```python
from build123d import *

# Parameters (mm, degrees)
SKETCH2_R                 = 203
BOSS_EXTRUDE1_DEPTH       = 25
SKETCH3_R                 = 165
BOSS_EXTRUDE4_DEPTH       = 20
BOSS_EXTRUDE6_DEPTH       = 45
BOSS_EXTRUDE7_DEPTH       = 202.626802206
SKETCH12_W                = 400
SKETCH12_H                = 84
CUT_EXTRUDE2_DEPTH        = 195
SKETCH13_R                = 65
BOSS_EXTRUDE8_DEPTH       = 5
SKETCH14_R                = 59.5
BOSS_EXTRUDE9_DEPTH       = 14
SKETCH15_R                = 21.046280496
BOSS_EXTRUDE10_DEPTH      = 14
BOSS_EXTRUDE11_DEPTH      = 25
BOSS_EXTRUDE12_DEPTH      = 65
BOSS_EXTRUDE12_DEPTH_BACK = 25
BOSS_EXTRUDE13_DEPTH      = 25
BOSS_EXTRUDE13_DEPTH_BACK = 15
FILLET1_R                 = 10
SKETCH20_R                = 116.015
BOSS_EXTRUDE14_DEPTH      = 10


with BuildPart() as part:
    # Sketch2 → Boss-Extrude1 (new body)
    with BuildSketch(Plane(origin=(0, 0, 0), x_dir=(1, 0, 0), z_dir=(0, 1, 0))):
        with Locations(Location((0, 0, 0), (0, 0, 270))):
            Circle(SKETCH2_R)
    extrude(amount=BOSS_EXTRUDE1_DEPTH)

    # Sketch3 → Boss-Extrude4 (add)
    with BuildSketch(Plane(origin=(0, 25, 0), x_dir=(1, 0, 0), z_dir=(0, 1, 0))):
        with Locations(Location((0, 0, 0), (0, 0, 270))):
            Circle(SKETCH3_R)
    extrude(amount=BOSS_EXTRUDE4_DEPTH)

    # Sketch8 → Boss-Extrude6 (add)
    with BuildSketch(Plane(origin=(0, 45, 0), x_dir=(1, 0, 0), z_dir=(0, 1, 0))):
        Polygon((-36.218523686, 88.373197794), (-36.218523686, 142.845857418), (-66.931831772, 173.559165504), (-278.448010099, 88.373197794), (-278.448010099, -114.626802206), (-36.218523686, -114.626802206), align=None)
    extrude(amount=-BOSS_EXTRUDE6_DEPTH)

    # Sketch11 → Boss-Extrude7 (add)
    with BuildSketch(Plane.XY.offset(-88)):
        Polygon((-278.448010099, 0), (-364.82630567, -41.890214301), (-773.82630567, -41.890214301), (-773.82630567, 82.109785699), (-433.530139449, 82.109785699), (-278.448010099, 45), align=None)
    extrude(amount=BOSS_EXTRUDE7_DEPTH)

    # Sketch12 → Cut-Extrude2 (cut)
    with BuildSketch(Plane(origin=(0, 0, -88), x_dir=(-1, 0, 0), z_dir=(0, 0, -1))):
        with Locations((573.82630567, 20.109785699)):
            Rectangle(SKETCH12_W, SKETCH12_H)
    extrude(amount=-CUT_EXTRUDE2_DEPTH, mode=Mode.SUBTRACT)

    # Sketch13 → Boss-Extrude8 (add)
    with BuildSketch(Plane.XZ.offset(41.890214301)):
        with Locations((-572.873962689, 13.972710812)):
            Circle(SKETCH13_R)
    extrude(amount=BOSS_EXTRUDE8_DEPTH)

    # Sketch14 → Boss-Extrude9 (add)
    with BuildSketch(Plane.XZ.offset(46.890214301)):
        with Locations((-572.873962689, 13.972710812)):
            Circle(SKETCH14_R)
    extrude(amount=BOSS_EXTRUDE9_DEPTH)

    # Sketch15 → Boss-Extrude10 (add)
    with BuildSketch(Plane(origin=(0, 82.109785699, 0), x_dir=(1, 0, 0), z_dir=(0, 1, 0))):
        with Locations(Location((-702.441522293, -14.627430099, 0), (0, 0, 90))):
            Circle(SKETCH15_R)
        with Locations(Location((-628.892568706, -14.627430099, 0), (0, 0, 90))):
            Circle(SKETCH15_R)
        with Locations(Location((-572.1226233, -14.627430099, 0), (0, 0, 90))):
            Circle(SKETCH15_R)
    extrude(amount=BOSS_EXTRUDE10_DEPTH)

    # Sketch16 → Boss-Extrude11 (add)
    with BuildSketch(Plane(origin=(0, 96.109785699, 0), x_dir=(1, 0, 0), z_dir=(0, 1, 0))):
        with BuildLine():
            Line((-556.497428598, 64.069909455), (-974.176536307, 64.069909455))
            Line((-974.176536307, 64.069909455), (-1038.149417409, 0.097028353))
            ThreePointArc((-1038.149417409, 0.097028353), (-1064.162147568, -38.833773506), (-1073.296603667, -84.75578539))
            Line((-1073.296603667, -84.75578539), (-1073.296603667, -142.077234659))
            ThreePointArc((-1073.296603667, -142.077234659), (-1038.149417409, -226.930048402), (-953.296603667, -262.077234659))
            Line((-953.296603667, -262.077234659), (-636.497428598, -262.077234659))
            ThreePointArc((-636.497428598, -262.077234659), (-551.644614856, -226.930048402), (-516.497428598, -142.077234659))
            Line((-516.497428598, -142.077234659), (-516.497428598, 24.069909455))
            ThreePointArc((-516.497428598, 24.069909455), (-528.213157351, 52.354180702), (-556.497428598, 64.069909455))
        make_face()
    extrude(amount=BOSS_EXTRUDE11_DEPTH)

    # Sketch17 → Boss-Extrude12 (add, two sides: drawn at the far end of the back side and taken through both)
    with BuildSketch(Plane.ZY.offset(1073.296603667).offset(-BOSS_EXTRUDE12_DEPTH_BACK)):
        with BuildLine():
            Line((8.768612392, 544.923564191), (123.173449264, 544.923564191))
            ThreePointArc((123.173449264, 544.923564191), (222.16839863, 503.918513558), (263.173449264, 404.923564191))
            Line((263.173449264, 404.923564191), (263.173449264, -54.759891123))
            ThreePointArc((263.173449264, -54.759891123), (222.16839863, -153.754840489), (123.173449264, -194.759891123))
            Line((123.173449264, -194.759891123), (8.768612392, -194.759891123))
            ThreePointArc((8.768612392, -194.759891123), (-90.226336974, -153.754840489), (-131.231387608, -54.759891123))
            Line((-131.231387608, -54.759891123), (-131.231387608, 404.923564191))
            ThreePointArc((-131.231387608, 404.923564191), (-90.226336974, 503.918513558), (8.768612392, 544.923564191))
        make_face()
    extrude(amount=BOSS_EXTRUDE12_DEPTH + BOSS_EXTRUDE12_DEPTH_BACK)

    # Sketch19 → Boss-Extrude13 (add, two sides: drawn at the far end of the back side and taken through both)
    with BuildSketch(Plane(origin=(0, 0, -23.231387608), x_dir=(-1, 0, 0), z_dir=(0, 0, -1)).offset(-BOSS_EXTRUDE13_DEPTH_BACK)):
        Polygon((1052.931156926, -16.752524753), (985.063520649, 100.43883668), (1052.931156926, 100.43883668), align=None)
    extrude(amount=BOSS_EXTRUDE13_DEPTH + BOSS_EXTRUDE13_DEPTH_BACK)

    # Fillet1
    fillet1_edges = [part.edges().sort_by_distance(p)[0] for p in [
        (-1048.296603667, -8.749747053, -28.231387608),
        (-987.570552343, 96.109785699, -28.231387608),
    ]]
    fillet(fillet1_edges, radius=FILLET1_R)

    # Sketch20 → Boss-Extrude14 (add)
    with BuildSketch(Plane(origin=(-1048.296603667, 0, 0), x_dir=(0, 0, -1), z_dir=(1, 0, 0))):
        with Locations(Location((-39.49671875, 302.878292984, 0), (0, 0, 270))):
            Circle(SKETCH20_R)
    extrude(amount=BOSS_EXTRUDE14_DEPTH)


solid = part.part
```
The model under review builds one solid part; all positions refer to its coordinate system, in mm. A direction names the side the tool comes from. Round coordinates to 2 decimals unless told otherwise and drop trailing zeros. Loops run counter-clockwise (first coordinate to the right, second up) from the corner with the lowest first, then second, coordinate; pieces in that order, holes last. Notation, with made-up numbers: M 42.25,1 L 47.25,1 A24 cw 47.25,19 Z; hole C -1.5,64.5 d10. An arc over 180 degrees is marked long. Answer as a JSON object with one key per item and string values.
(1) Clearance check with flat-ended pins moving along their axes: P1, Ø20, axis at x = -806, y = 108, coming from the +Z side; P2, Ø8, axis at y = -91.5, z = 145, coming from the +X side; P3, Ø12.5, axis at y = 110, z = 59, coming from the +X side. State where each tip first meets the part, or that it passes through.
Resolved:
{"P1": "z = 262.08", "P2": "x = -1048.3", "P3": "x = -516.5"}
(2) Take a section at D-D on x = -815.5. Give the boundary of the cut face in (y, z).
Resolved:
{"outline": "M 96.11,-64.07 L 121.11,-64.07 L 121.11,262.08 L 96.11,262.08 Z"}
(3) Take a section at B-B on z = 233. Give the boundary of the cut face in (x, y), and give its area (3 significant figures).
Resolved:
{"outline": "M -1138.3,-141.58 L -1048.3,-141.58 L -1048.3,491.75 L -1138.3,491.75 Z; M -1031.61,96.11 L -558.18,96.11 L -558.18,121.11 L -1031.61,121.11 Z", "area": "68,800 mm²"}
(4) Take a section at A-A on x = 0. Give the boundary of the cut face in (y, z).
Resolved:
{"outline": "M 0,-203 L 25,-203 L 25,-165 L 45,-165 L 45,165 L 25,165 L 25,203 L 0,203 Z"}
(5) To check wall thickness, follow line 1 along Y through (x, z) = (-706.5, -62); line 2 along Y through (x, z) = (-713, 208); line 3 along X through (y, z) = (85, 219). State the ranges of each line that lie inside material, in increasing order.
Resolved:
{"line 1": "-41.89 to -21.89, 62.11 to 82.11, 96.11 to 121.11", "line 2": "96.11 to 121.11", "line 3": "-1138.3 to -1048.3"}
(6) Draft analysis for pull direction X (two halves, no side actions). For faces 6 (the flat face through (-516.497, 108, 60)), 7 (the flat face through (-467.6, 62.3, -88)), 8 (the flat face through (-1138.297, 180, 69)), 9 (the cylindrical face through (-608.347, 89.012, 19.19)), state which applies: released by +X, released by -X, zero draft, split by the parting line, or undercut.
Resolved:
{"face 6": "released by +X", "face 7": "undercut", "face 8": "released by -X", "face 9": "undercut"}
(7) Tool access review of faces 1 (the flat face through (-571, 62.11, 8)), 2 (the cylindrical face through (-592.99, 89.01, 17.37)), 3 (the flat face through (-1038.297, 305, 38)), 4 (the cylindrical face through (-516.12, -53.79, 31.84)), 5 (the cylindrical face through (158.766, 34.86, 44.926)): name each direction out of +Z, -Z, +X, -X, +Y, -Y from which nothing blocks a thin tool from reaching the whole face with its end or side.
Resolved:
{"face 1": "-Z", "face 2": "none", "face 3": "+Z, -Z, +X, +Y", "face 4": "-Y", "face 5": "+Y"}
(8) Take a section at C-C on y = 205. Give the boundary of the cut face in (x, z).
Resolved:
{"outline": "M -1138.3,-131.23 L -1048.3,-131.23 L -1048.3,-22.79 L -1038.3,-22.79 L -1038.3,101.78 L -1048.3,101.78 L -1048.3,263.17 L -1138.3,263.17 Z"}
